Verification items for this drawing (mm, ordinates from the low corner). Round coordinates to 2 decimals unless told otherwise and drop trailing zeros. Loops run counter-clockwise (first coordinate to the right, second up) from the corner with the lowest first, then second, coordinate; pieces in that order, holes last. Notation, with made-up numbers: M 15.5,76 L 66.5,76 A22 ccw 66.5,95 Z; hole C 18,-1.5 d9. An arc over 180 degrees is marked long. Write item = value, one per line. Start each with the question number.
(1) Cross-section at A-A on z = 2.15. Record the boundary of the cut face in (x, y).
(2) Cross-section at C-C on x = 30. Record the boundary of the cut face in (y, z).
(3) Scan lines: L1, parallel to X at y = 42, z = 4.8; L2, parallel to Y at x = 7, z = 0.5. Record each from-to range of solid material in increasing order. Write a range as from..to.
(4) Go/stop test with flat-tipped pins: P1, Ø2.5, axis at y = 116, z = 3.5, coming from the -X side; P2, Ø1.5, axis at x = 8.5, z = 1.5, coming from the -Y side; P3, Ø2.5, axis at x = 1.5, z = 3.5, coming from the -Y side. Record where each tip stops, or that it passes through.
(5) Cross-section at B-B on y = 151. Record the boundary of the cut face in (x, z).
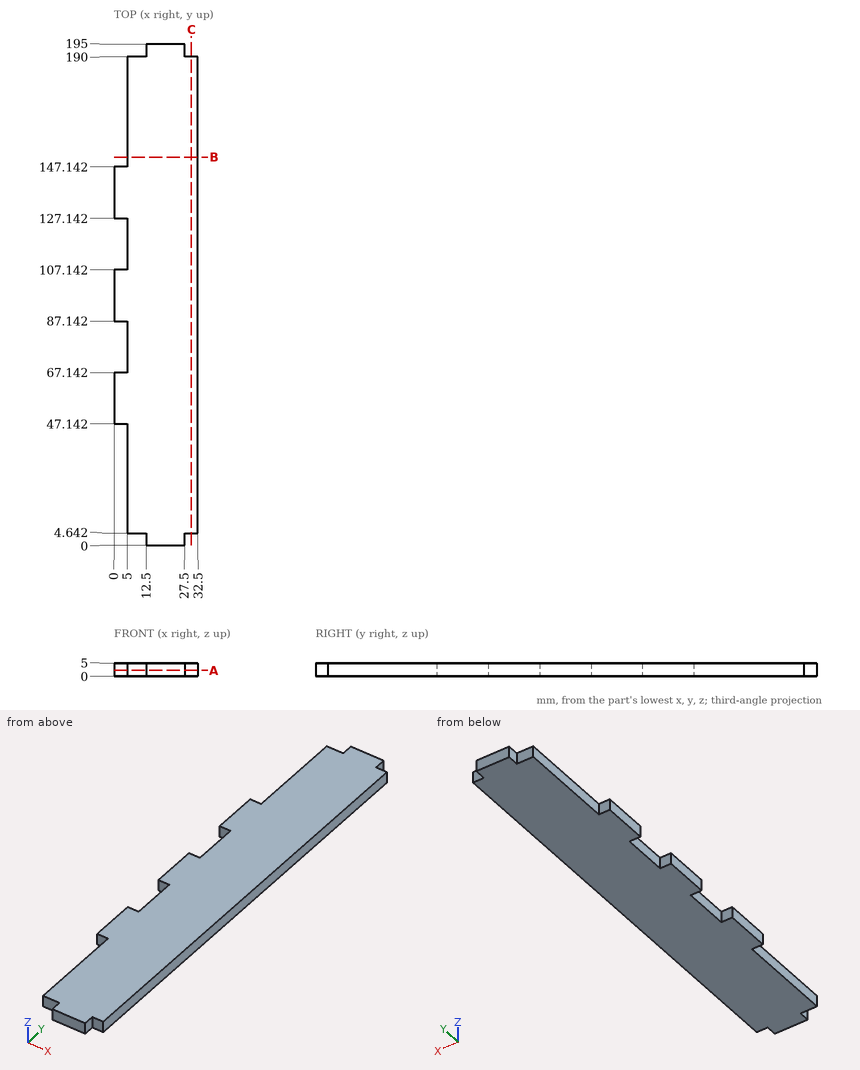
Result:
q1.outline = M 0,47.14 L 5,47.14 L 5,4.64 L 12.5,4.64 L 12.5,0 L 27.5,0 L 27.5,4.64 L 32.5,4.64 L 32.5,190 L 27.5,190 L 27.5,195 L 12.5,195 L 12.5,190 L 5,190 L 5,147.14 L 0,147.14 L 0,127.14 L 5,127.14 L 5,107.14 L 0,107.14 L 0,87.14 L 5,87.14 L 5,67.14 L 0,67.14 Z
q2.outline = M 4.64,0 L 190,0 L 190,5 L 4.64,5 Z
q3.L1 = 5..32.5
q3.L2 = 4.64..190
q4.P1 = 5
q4.P2 = 4.64
q4.P3 = 47.14
q5.outline = M 5,0 L 32.5,0 L 32.5,5 L 5,5 Z
